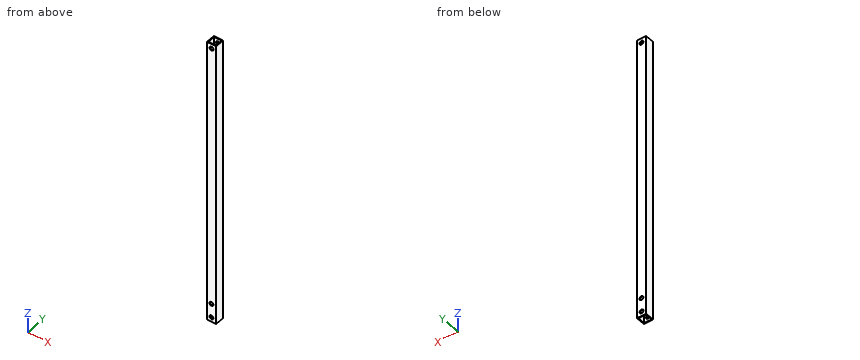
```python
from build123d import *

# Parameters (mm, degrees)
SKETCH_2_W          = 10
SKETCH_2_H          = 10
SKETCH_2_W_2        = 8
SKETCH_2_H_2        = 8
EXTRUDE_1_DEPTH     = 310
CUT_EXTRUDE_1_REACH = 312.322
SKETCH_3_R          = 2.15


with BuildPart() as part:
    # ｽｹｯﾁ2 → 押し出し-薄板1 (new body)
    with BuildSketch(Plane.XY):
        with Locations((5, 5)):
            Rectangle(SKETCH_2_W, SKETCH_2_H)
        with Locations((5, 5)):
            Rectangle(SKETCH_2_W_2, SKETCH_2_H_2, mode=Mode.SUBTRACT)
    extrude(amount=EXTRUDE_1_DEPTH)

    # ｶｯﾄ - 押し出し1: up to this face of the body (flat: up to its plane)
    cut_extrude_1_end = Plane(part.part.faces().sort_by_distance((5, 0, 155))[0])
    # ｽｹｯﾁ3 → ｶｯﾄ - 押し出し1 (cut, up to the picked face)
    with BuildSketch(Plane(origin=(0, 10, 0), x_dir=(1, 0, 0), z_dir=(0, 1, 0)), mode=Mode.PRIVATE) as cut_extrude_1_sk1:
        with Locations(Location((5, -305, 0), (0, 0, 270))):
            Circle(SKETCH_3_R)
    cut_extrude_1_tool1 = split(extrude(cut_extrude_1_sk1.sketch, amount=-CUT_EXTRUDE_1_REACH, mode=Mode.PRIVATE), bisect_by=cut_extrude_1_end, keep=Keep.BOTH, mode=Mode.PRIVATE)
    # ｽｹｯﾁ3 → ｶｯﾄ - 押し出し1 (cut, up to the picked face)
    with BuildSketch(Plane(origin=(0, 10, 0), x_dir=(1, 0, 0), z_dir=(0, 1, 0)), mode=Mode.PRIVATE) as cut_extrude_1_sk2:
        with Locations(Location((5, -5, 0), (0, 0, 90))):
            Circle(SKETCH_3_R)
    cut_extrude_1_tool2 = split(extrude(cut_extrude_1_sk2.sketch, amount=-CUT_EXTRUDE_1_REACH, mode=Mode.PRIVATE), bisect_by=cut_extrude_1_end, keep=Keep.BOTH, mode=Mode.PRIVATE)
    # ｽｹｯﾁ3 → ｶｯﾄ - 押し出し1 (cut, up to the picked face)
    with BuildSketch(Plane(origin=(0, 10, 0), x_dir=(1, 0, 0), z_dir=(0, 1, 0)), mode=Mode.PRIVATE) as cut_extrude_1_sk3:
        with Locations(Location((5, -20, 0), (0, 0, 270))):
            Circle(SKETCH_3_R)
    cut_extrude_1_tool3 = split(extrude(cut_extrude_1_sk3.sketch, amount=-CUT_EXTRUDE_1_REACH, mode=Mode.PRIVATE), bisect_by=cut_extrude_1_end, keep=Keep.BOTH, mode=Mode.PRIVATE)
    add(cut_extrude_1_tool1.solids().sort_by(Axis((5, 10, 305), (0, -1, 0)))[0], mode=Mode.SUBTRACT)
    add(cut_extrude_1_tool2.solids().sort_by(Axis((5, 10, 5), (0, -1, 0)))[0], mode=Mode.SUBTRACT)
    add(cut_extrude_1_tool3.solids().sort_by(Axis((5, 10, 20), (0, -1, 0)))[0], mode=Mode.SUBTRACT)


solid = part.part
```
The listing builds one solid part. Answer for the finished solid, in the listing's coordinates (mm). Give positions to 0.01 mm unless a question says otherwise; leave off trailing zeros. Loops run counter-clockwise (first coordinate to the right, second up) from the corner with the lowest first, then second, coordinate; pieces in that order, holes last. Notation, with made-up numbers: (-30, 77) - (-4, 77) arc R35 cw to (-4, 111) - close; hole circle Ø5 at (-4, 11). An arc over 180 degrees is marked (long way). Return JSON: item names as keys, results as strings. Group by question number.
1. Given pin 1 Ø2.5 at (x, z) = (5, 20) entering from -Y, flat-ended and moving along its own axis, determine where the tip first touches the part or whether it passes through.
2. Find section C-C (y = 5.75). Write down the section's boundary in (x, z).
3. Find section A-A (x = 5). State how many separate pieces and enclosed holes the cut face has, then the cut area to 3 significant figures.
4. Find section B-B (z = 55). Write down the section's boundary in (x, y), then the cut area to 3 significant figures.
5. Straight lines are drawn through the part: line 1 (Y direction, x = 4.5, z = 239); line 2 (X direction, y = 9.75, z = 5). For each, find the intervals that lie inside material, in ascending order. Write a range as [from, to].
Verdict:
{
 "1": {"pin 1": "passes through"},
 "2": {"outline": "(0, 0) - (1, 0) - (1, 310) - (0, 310) - close; (9, 0) - (10, 0) - (10, 310) - (9, 310) - close"},
 "3": {"separate pieces": "8", "enclosed holes": "0", "area": "594 mm^2"},
 "4": {"outline": "(0, 0) - (10, 0) - (10, 10) - (0, 10) - close; hole (1, 1) - (9, 1) - (9, 9) - (1, 9) - close", "area": "36.0 mm^2"},
 "5": {"line 1": "y = [0, 1], [9, 10]", "line 2": "x = [0, 2.85], [7.15, 10]"}
}
